from build123d import *

# Parameters (mm, degrees)
ESQUISSE1_W                       = 320
ESQUISSE1_H                       = 320
BOSS_EXTRU_1_DEPTH                = 3
ENL_V_MAT_EXTRU_1_REACH           = 5
ESQUISSE2_W                       = 60
ESQUISSE2_H                       = 60
ESQUISSE3_W                       = 202
ESQUISSE3_H                       = 202
ESQUISSE3_W_2                     = 198
ESQUISSE3_H_2                     = 198
ENL_V_MAT_EXTRU_2_DEPTH           = 1
DIAM_TRE_DU_PER_AGE_5_0_5_1_D     = 5
DIAM_TRE_DU_PER_AGE_5_0_5_1_DEPTH = 3


with BuildPart() as part:
    # Esquisse1 → Boss.-Extru.1 (new body)
    with BuildSketch(Plane.XY):
        Rectangle(ESQUISSE1_W, ESQUISSE1_H)
    extrude(amount=BOSS_EXTRU_1_DEPTH)

    # Esquisse2 → Enlèv. mat.-Extru.1 (cut, up to next)
    with BuildSketch(Plane.XY.offset(3), mode=Mode.PRIVATE) as enl_v_mat_extru_1_sk1:
        with Locations((130, -130)):
            Rectangle(ESQUISSE2_W, ESQUISSE2_H)
    enl_v_mat_extru_1_tool1 = extrude(enl_v_mat_extru_1_sk1.sketch, amount=-ENL_V_MAT_EXTRU_1_REACH, mode=Mode.PRIVATE) & part.part
    add(enl_v_mat_extru_1_tool1.solids().sort_by_distance((130, -130, 3))[0], mode=Mode.SUBTRACT)
    # Esquisse2 → Enlèv. mat.-Extru.1 (cut, up to next)
    with BuildSketch(Plane.XY.offset(3), mode=Mode.PRIVATE) as enl_v_mat_extru_1_sk2:
        with Locations((-130, -130)):
            Rectangle(ESQUISSE2_W, ESQUISSE2_H)
    enl_v_mat_extru_1_tool2 = extrude(enl_v_mat_extru_1_sk2.sketch, amount=-ENL_V_MAT_EXTRU_1_REACH, mode=Mode.PRIVATE) & part.part
    add(enl_v_mat_extru_1_tool2.solids().sort_by_distance((-130, -130, 3))[0], mode=Mode.SUBTRACT)
    # Esquisse2 → Enlèv. mat.-Extru.1 (cut, up to next)
    with BuildSketch(Plane.XY.offset(3), mode=Mode.PRIVATE) as enl_v_mat_extru_1_sk3:
        with Locations((130, 130)):
            Rectangle(ESQUISSE2_W, ESQUISSE2_H)
    enl_v_mat_extru_1_tool3 = extrude(enl_v_mat_extru_1_sk3.sketch, amount=-ENL_V_MAT_EXTRU_1_REACH, mode=Mode.PRIVATE) & part.part
    add(enl_v_mat_extru_1_tool3.solids().sort_by_distance((130, 130, 3))[0], mode=Mode.SUBTRACT)
    # Esquisse2 → Enlèv. mat.-Extru.1 (cut, up to next)
    with BuildSketch(Plane.XY.offset(3), mode=Mode.PRIVATE) as enl_v_mat_extru_1_sk4:
        with Locations((-130, 130)):
            Rectangle(ESQUISSE2_W, ESQUISSE2_H)
    enl_v_mat_extru_1_tool4 = extrude(enl_v_mat_extru_1_sk4.sketch, amount=-ENL_V_MAT_EXTRU_1_REACH, mode=Mode.PRIVATE) & part.part
    add(enl_v_mat_extru_1_tool4.solids().sort_by_distance((-130, 130, 3))[0], mode=Mode.SUBTRACT)

    # Esquisse3 → Enlèv. mat.-Extru.2 (cut)
    with BuildSketch(Plane.XY.offset(3)):
        Rectangle(ESQUISSE3_W, ESQUISSE3_H)
        Rectangle(ESQUISSE3_W_2, ESQUISSE3_H_2, mode=Mode.SUBTRACT)
    extrude(amount=-ENL_V_MAT_EXTRU_2_DEPTH, mode=Mode.SUBTRACT)

    # Diamètre du perçage Ø5.0 (5)1
    with Locations(Plane.XY.offset(3)):
        with Locations((32.349968284, -30.166833461), (43.320273808, -40.396808862)):
            Hole(DIAM_TRE_DU_PER_AGE_5_0_5_1_D / 2, depth=DIAM_TRE_DU_PER_AGE_5_0_5_1_DEPTH)


solid = part.part
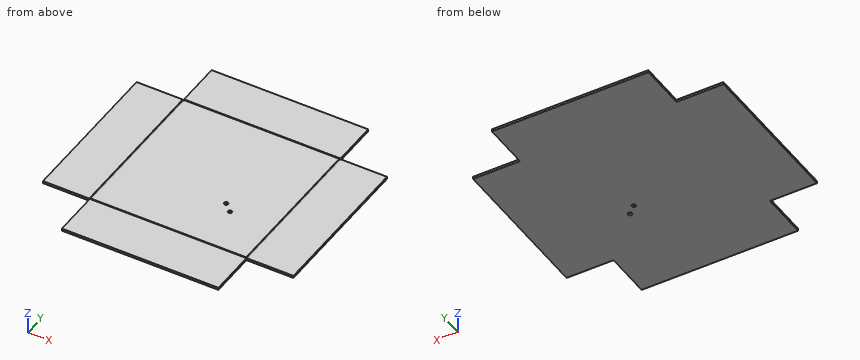
Could you check a few things on this model? Use its own coordinates, in mm. Coordinates: 2 decimals unless noted, no trailing zeros. Order: outer loops, then holes, each group sorted by start corner. A loop starts at its lowest first (then second) coordinate and runs counter-clockwise, first axis right, second up.
Q1. Will these pins go through, and if not, where does the flat tip stop? pin 1 (0.9 mm diameter, centred on y = 115, z = 1.5, fed in from -X); pin 2 (1 mm diameter, centred on x = 82, y = 99.5, fed in from -Z).
Q2. Suppose I cut it at B-B on x = 138.5. Please give me the cut outline in (y, z).
Q3. Suppose I cut it at A-A on z = 0.75. Please give me the cut outline in (x, y), and give its area (3 significant figures).
Q4. Please list where these lines run through material, in increasing order: L1, parallel to Y at x = 1, z = 2.9; L2, parallel to X at y = 113, z = 0.2.
Answer:
1. pin 1: stops at x = -100
1. pin 2: stops at z = 0
2. outline: (-100, 0) - (100, 0) - (100, 3) - (-100, 3) - close
3. outline: (-160, -100) - (-100, -100) - (-100, -160) - (100, -160) - (100, -100) - (160, -100) - (160, 100) - (100, 100) - (100, 160) - (-100, 160) - (-100, 100) - (-160, 100) - close; hole circle Ø5 at (32.35, -30.17); hole circle Ø5 at (43.32, -40.4)
3. area: 88,000 mm2
4. L1: y = -160 to -101, -99 to 99, 101 to 160
4. L2: x = -100 to 100
